The figure shows three views and two pictorial views of one solid part (mm, origin at its lowest corner). Answer the questions. A direction names the side the tool comes from. Round coordinates to 2 decimals unless told otherwise and drop trailing zeros. Order: outer loops, then holes, each group sorted by start corner. A loop starts at its lowest first (then second) coordinate and runs counter-clockwise, first axis right, second up. Notation, with made-up numbers: (-5, 63) - (17, 63) arc R25 cw to (17, 101) - close; hole circle Ø9 at (17.25, -22.5). An arc over 180 degrees is marked (long way). Write item = value, one per line.
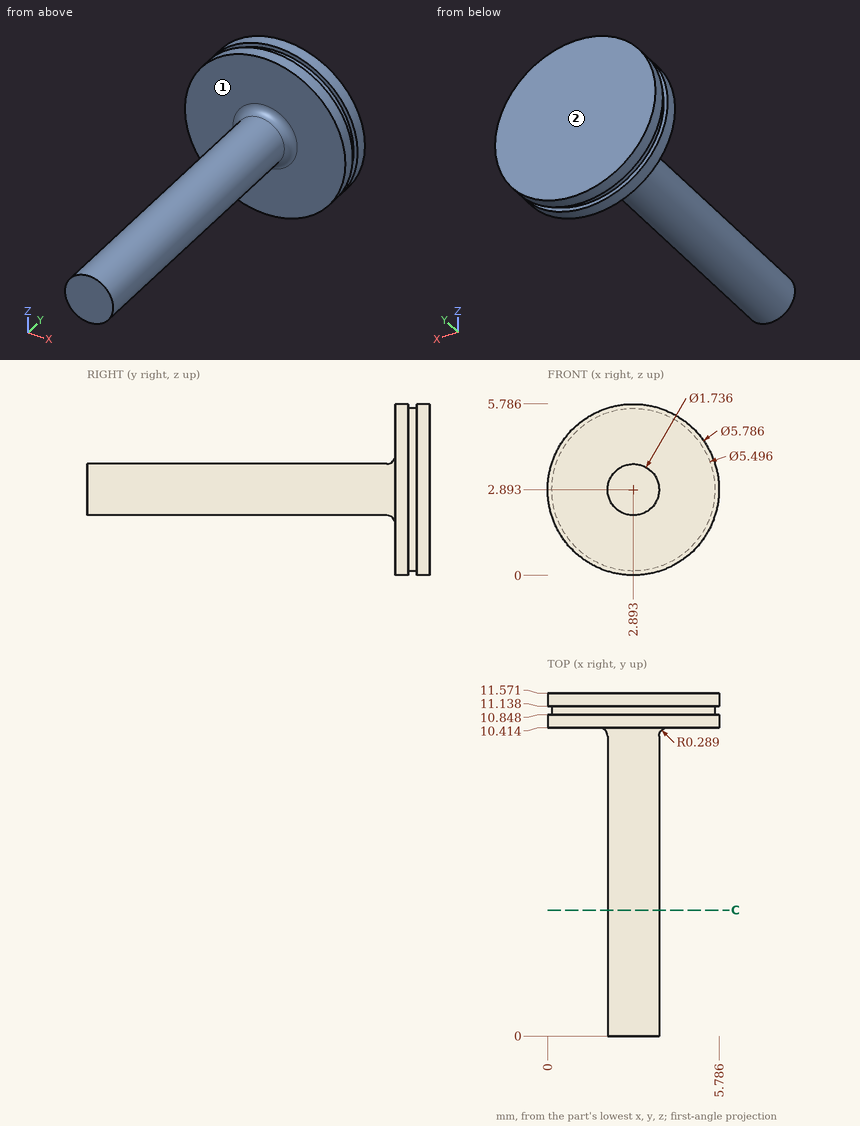
Q1. Flat-ended cylindrical pins translate along their axes: P1, Ø3, axis at y = 3, z = 2.5, coming from the -X side (1 decimal); P2, Ø2, axis at x = 4.5, y = 8, coming from the +Z side. Find the tip coordinate at first contact, or state that the pin passes through.
Model answer:
P1 = 2
P2 = 3.51
Q2. Section C-C on y = 4.25 is taken. Determine the outline of the cut face in (x, z) (1 decimal).
Model answer:
outline = circle Ø1.7 at (2.9, 2.9)
Q3. For the marked faces 1 and 2, determine the directions among +Z, -Z, +X, -X, +Y, -Y from which every point of the face is accessible in a straight line to the end or side of a thin tool.
Model answer:
face_1 = -Y
face_2 = +Z, -Z, +X, -X, +Y
Q4. Find the intervals of material crossed by line 1 (Y direction, x = 0.4, z = 1.6) (1 decimal); line 2 (Y direction, x = 3.25, z = 0.9) (1 decimal); line 3 (Z direction, x = 2.8, y = 10.75) (1 decimal), in increasing order. Write a range as from..to.
Model answer:
line_1 = 10.4..10.8, 11.1..11.6
line_2 = 10.4..11.6
line_3 = 0..5.8
